from build123d import *

# Parameters (mm, degrees)
F0_R     = 21.9
F0_R_2   = 16.35
F1_DEPTH = 0.8
F2_R     = 2
F2_W     = 5
F2_H     = 4.8
F2_W_2   = 4.8
F2_H_2   = 5
F3_DEPTH = 1.6
F4_DEPTH = 1.65
F6_DEPTH = 0.1


with BuildPart() as f1:
    # F0 (on Top) → F1 (new body)
    with BuildSketch(Plane.XY):
        Circle(F0_R)
        Circle(F0_R_2, mode=Mode.SUBTRACT)
    extrude(amount=F1_DEPTH)

    # F2 (on face) → F3 (join)
    with BuildSketch(Plane.XY.offset(0.8)):
        with BuildLine():
            Line((2.4, 21.625), (0, 21.625))
            Line((0, 21.625), (0, 21.125))
            ThreePointArc((0, 21.125), (1.4142135624, 20.5392135624), (2, 19.125))
            ThreePointArc((2, 19.125), (1.4142135624, 17.7107864376), (0, 17.125))
            Line((0, 17.125), (0, 16.625))
            Line((0, 16.625), (2.4, 16.625))
            Line((2.4, 16.625), (2.4, 21.625))
        make_face()
        with BuildLine():
            Line((0, 21.125), (0, 21.625))
            Line((0, 21.625), (-2.4, 21.625))
            Line((-2.4, 21.625), (-2.4, 16.625))
            Line((-2.4, 16.625), (0, 16.625))
            Line((0, 16.625), (0, 17.125))
            ThreePointArc((0, 17.125), (-2, 19.125), (0, 21.125))
        make_face()
        Polygon((-10.4928401029, 19.0604546529), (-8.5794229411, 14.4410569903), (-4.144801185, 16.2779374657), (-6.0582183469, 20.8973351282), align=None)
        with Locations((-7.318820644, 17.6691960593)):
            Circle(F2_R, mode=Mode.SUBTRACT)
        Polygon((-16.988240418, 13.5941278683), (-13.4527065121, 10.0585939624), (-10.0585939624, 13.4527065121), (-13.5941278683, 16.988240418), align=None)
        with Locations((-13.5234171902, 13.5234171902)):
            Circle(F2_R, mode=Mode.SUBTRACT)
        Polygon((-20.8973351282, 6.0582183469), (-16.2779374657, 4.144801185), (-14.4410569903, 8.5794229411), (-19.0604546529, 10.4928401029), align=None)
        with Locations((-17.6691960593, 7.318820644)):
            Circle(F2_R, mode=Mode.SUBTRACT)
        with Locations((-19.125, 0)):
            Rectangle(F2_W, F2_H)
        with Locations((-19.125, 0)):
            Circle(F2_R, mode=Mode.SUBTRACT)
        Polygon((-19.0604546529, -10.4928401029), (-14.4410569903, -8.5794229411), (-16.2779374657, -4.144801185), (-20.8973351282, -6.0582183469), align=None)
        with Locations((-17.6691960593, -7.318820644)):
            Circle(F2_R, mode=Mode.SUBTRACT)
        Polygon((-13.5941278683, -16.988240418), (-10.0585939624, -13.4527065121), (-13.4527065121, -10.0585939624), (-16.988240418, -13.5941278683), align=None)
        with Locations((-13.5234171902, -13.5234171902)):
            Circle(F2_R, mode=Mode.SUBTRACT)
        Polygon((-6.0582183469, -20.8973351282), (-4.144801185, -16.2779374657), (-8.5794229411, -14.4410569903), (-10.4928401029, -19.0604546529), align=None)
        with Locations((-7.318820644, -17.6691960593)):
            Circle(F2_R, mode=Mode.SUBTRACT)
        with Locations((0, -19.125)):
            Rectangle(F2_W_2, F2_H_2)
        with Locations((0, -19.125)):
            Circle(F2_R, mode=Mode.SUBTRACT)
        Polygon((10.4928401029, -19.0604546529), (8.5794229411, -14.4410569903), (4.144801185, -16.2779374657), (6.0582183469, -20.8973351282), align=None)
        with Locations((7.318820644, -17.6691960593)):
            Circle(F2_R, mode=Mode.SUBTRACT)
        Polygon((16.988240418, -13.5941278683), (13.4527065121, -10.0585939624), (10.0585939624, -13.4527065121), (13.5941278683, -16.988240418), align=None)
        with Locations((13.5234171902, -13.5234171902)):
            Circle(F2_R, mode=Mode.SUBTRACT)
        Polygon((20.8973351282, -6.0582183469), (16.2779374657, -4.144801185), (14.4410569903, -8.5794229411), (19.0604546529, -10.4928401029), align=None)
        with Locations((17.6691960593, -7.318820644)):
            Circle(F2_R, mode=Mode.SUBTRACT)
        with Locations((19.125, 0)):
            Rectangle(F2_W, F2_H)
        with Locations((19.125, 0)):
            Circle(F2_R, mode=Mode.SUBTRACT)
        Polygon((19.0604546529, 10.4928401029), (14.4410569903, 8.5794229411), (16.2779374657, 4.144801185), (20.8973351282, 6.0582183469), align=None)
        with Locations((17.6691960593, 7.318820644)):
            Circle(F2_R, mode=Mode.SUBTRACT)
        Polygon((13.5941278683, 16.988240418), (10.0585939624, 13.4527065121), (13.4527065121, 10.0585939624), (16.988240418, 13.5941278683), align=None)
        with Locations((13.5234171902, 13.5234171902)):
            Circle(F2_R, mode=Mode.SUBTRACT)
        Polygon((6.0582183469, 20.8973351282), (4.144801185, 16.2779374657), (8.5794229411, 14.4410569903), (10.4928401029, 19.0604546529), align=None)
        with Locations((7.318820644, 17.6691960593)):
            Circle(F2_R, mode=Mode.SUBTRACT)
    extrude(amount=F3_DEPTH)

    # F4 (add): faces of the model
    f4_faces = [f1.faces().sort_by_distance(p)[0] for p in [
        (-17.6691960593, 7.318820644, 0.8),
        (-13.5234171902, 13.5234171902, 0.8),
        (-7.318820644, 17.6691960593, 0.8),
        (0, 19.125, 0.8),
        (7.318820644, 17.6691960593, 0.8),
        (-19.125, 0, 0.8),
        (-17.6691960593, -7.318820644, 0.8),
        (-13.5234171902, -13.5234171902, 0.8),
        (-7.318820644, -17.6691960593, 0.8),
        (0, -19.125, 0.8),
        (7.318820644, -17.6691960593, 0.8),
        (13.5234171902, -13.5234171902, 0.8),
        (17.6691960593, -7.318820644, 0.8),
        (19.125, 0, 0.8),
        (13.5234171902, 13.5234171902, 0.8),
        (17.6691960593, 7.318820644, 0.8),
    ]]
    extrude(f4_faces, amount=F4_DEPTH)

    # F5 (on face) → F6 (join)
    with BuildSketch(Plane(origin=(0, 0, 0), x_dir=(1, 0, 0), z_dir=(0, 0, -1))):
        Polygon((7.557822985, 19.3773058048), (6.4165551654, 19.748126198), (5.4895041823, 16.8949566491), (6.6307720019, 16.5241362559), align=None)
        Polygon((1.9239364053, 20.7098801839), (0.7246674128, 20.75175958), (0.6199689227, 17.7535870989), (1.8192379152, 17.7117077029), align=None)
        Polygon((4.7874710341, 20.240572858), (3.6057017305, 20.4489506712), (3.0847571975, 17.4945274122), (4.2665265011, 17.286149599), align=None)
        Polygon((-0.6199689227, 17.7535870989), (-0.7246674128, 20.75175958), (-1.9239364053, 20.7098801839), (-1.8192379152, 17.7117077029), align=None)
        Polygon((-3.0847571975, 17.4945274122), (-3.6057017305, 20.4489506712), (-4.7874710341, 20.240572858), (-4.2665265011, 17.286149599), align=None)
        Polygon((-5.4895041823, 16.8949566491), (-6.4165551654, 19.748126198), (-7.557822985, 19.3773058048), (-6.6307720019, 16.5241362559), align=None)
    extrude(amount=F6_DEPTH)


solid = f1.part
Could you check a few things on this model? Use its own coordinates, in mm. A direction names the side the tool comes from. Coordinates: 2 decimals unless noted, no trailing zeros. Write each loop counter-clockwise with the first axis right and the second up, starting at its lowest first coordinate (ties: lowest second). Pieces come first, ordered by that corner, then holes. Notation, with made-up numbers: (75.5, 43.25) - (96.5, 43.25) arc R37 ccw to (96.5, 81.25) - close; hole circle Ø3 at (85, 3). An arc over 180 degrees is marked (long way). Write item = value, one per line.
1) Suppose I cut it at A-A on y = 0. Please give me the cut outline in (x, z) (3 decimals), plus the area to 3 significant figures.
Result set:
outline = (-21.9, 0) - (-16.35, 0) - (-16.35, 0.8) - (-16.625, 0.8) - (-16.625, 2.4) - (-17.125, 2.4) - (-17.125, 2.45) - (-21.125, 2.45) - (-21.125, 2.4) - (-21.625, 2.4) - (-21.625, 0.8) - (-21.9, 0.8) - close; (16.35, 0) - (21.9, 0) - (21.9, 0.8) - (21.625, 0.8) - (21.625, 2.4) - (21.125, 2.4) - (21.125, 2.45) - (17.125, 2.45) - (17.125, 2.4) - (16.625, 2.4) - (16.625, 0.8) - (16.35, 0.8) - close
area = 25.3 mm2
2) We'd pull the mould along Y, two halves only. Please class faces 1 (the flat face through (8.307, 19.966, 1.589)), 2 (the flat face through (-9, 16, 2.4)), 3 (the cylindrical face through (-17.4, -13.3, 0.4)): +Y half, -Y half, draft (parallel to the pull), parting line (faces both ways), or undercut.
Result set:
face_1 = +Y half
face_2 = undercut
face_3 = parting line
3) Suppose I cut it at C-C on y = -8. Please give me the cut outline in (x, z), plus the area to 3 significant figures.
Result set:
outline = (-20.39, 0) - (-14.26, 0) - (-14.26, 0.8) - (-14.68, 0.8) - (-14.68, 2.4) - (-15.79, 2.4) - (-15.79, 2.45) - (-19.55, 2.45) - (-19.55, 2.4) - (-20.09, 2.4) - (-20.09, 0.8) - (-20.39, 0.8) - close; (14.26, 0) - (20.39, 0) - (20.39, 0.8) - (20.09, 0.8) - (20.09, 2.4) - (19.55, 2.4) - (19.55, 2.45) - (15.79, 2.45) - (15.79, 2.4) - (14.68, 2.4) - (14.68, 0.8) - (14.26, 0.8) - close
area = 27.5 mm2
4) Suppose I cut it at B-B on z = 2. State how many separate pieces and enclosed holes the cut face has, plus the area to 3 significant figures.
Result set:
separate_pieces = 16
enclosed_holes = 0
area = 384 mm2
5) Will these pins go through, and if not, where does the flat tip stop? pin 1 Ø0.5 at (y, z) = (19, 1.5) entering from -X; pin 2 Ø2 at (x, y) = (0.5, 14) entering from +Z; pin 3 Ø1.5 at (x, y) = (11, -15) entering from +Z; pin 4 Ø1.5 at (x, z) = (3.5, 2) entering from +Y.
Result set:
pin_1 = -10.49
pin_2 = through
pin_3 = 2.4
pin_4 = 16.53
6) Please list where these lines run through material, in increasing order: line 1 (Y direction, x = 0, z = 0.4); line 2 (X direction, y = 15, z = 0.9); line 3 (X direction, y = 0, z = 1.1) (3 decimals). Write a range as [from, to].
Result set:
line_1 = [-21.9, -16.35], [16.35, 21.9]
line_2 = [-15.58, -11.61], [-8.81, -7.23], [7.23, 8.81], [11.61, 15.58]
line_3 = [-21.625, -16.625], [16.625, 21.625]
7) For faces 4 (the flat face through (15.27, -15.31, 1.59)), 5 (the flat face through (19.992, 8.244, 1.589)), 6 (the flat face through (-5.115, -18.62, 1.589)), which set-ups out of +Z, -Z, +X, -X, +Y, -Y let a thin tool reach every point of the face, with its end or its side?
Result set:
face_4 = +Z, +X, -Y
face_5 = +Z, +X, +Y
face_6 = +Z, -Y
